```python
from build123d import *

# Parameters (mm, degrees)
SKETCH2_W  = 5.6
SKETCH2_H  = 1
SLOT_DEPTH = 0.7


with BuildPart() as part:
    # BodySke → Base-Revolve (revolve)
    with BuildSketch(Plane.XY):
        with BuildLine():
            Line((2.4, 1.5), (2.4, 2.8))
            Line((2.4, 2.8), (1.2, 2.8))
            ThreePointArc((1.2, 2.8), (0.351471863, 2.448528137), (0, 1.6))
            Line((0, 1.6), (0, 0))
            Line((0, 0), (8.4, 0))
            Line((8.4, 0), (8.4, 1.5))
            Line((8.4, 1.5), (2.4, 1.5))
        make_face()
    revolve(axis=Axis((-25.4, 0, 0), (1, 0, 0)))

    # Sketch2 → Slot (cut)
    with BuildSketch(Plane(origin=(0, 0, 0), x_dir=(0, 0, -1), z_dir=(1, 0, 0))):
        Rectangle(SKETCH2_W, SKETCH2_H)
    extrude(amount=SLOT_DEPTH, mode=Mode.SUBTRACT)


solid = part.part
```
Here's how the part is built. I have some questions about the finished solid (model axes, mm). A direction names the side the tool comes from. Round coordinates to 2 decimals unless told otherwise and drop trailing zeros. Loops run counter-clockwise (first coordinate to the right, second up) from the corner with the lowest first, then second, coordinate; pieces in that order, holes last.
1. Will these pins go through, and if not, where does the flat tip stop? pin 1 (2 mm diameter, centred on x = 3.5, z = 1, fed in from +Y); pin 2 (1.5 mm diameter, centred on y = -2, z = -1.5, fed in from +X); pin 3 (0.5 mm diameter, centred on y = 0, z = 1, fed in from -X).
Answers:
pin 1: stops at y = 1.5
pin 2: stops at x = 2.4
pin 3: stops at x = 0.7
2. Thinking about a two-plate mould opening in Y: for faces 1 (the face through (0, 1, 0)), 2 (the face through (1.8, -2.8, 0.1)), 3 (the face through (0.7, 0, 0)), which applies, released by +Y, released by -Y, zero draft, split by the parting line, or undercut?
Answers:
face 1: zero draft
face 2: split by the parting line
face 3: undercut
3. Suppose I cut it at B-B, the plane y = 0. Please give me the cut outline in (x, z).
Answers:
outline: (0.7, -2.69) arc R1.2 ccw to (1.2, -2.8) - (2.4, -2.8) - (2.4, -1.5) - (8.4, -1.5) - (8.4, 1.5) - (2.4, 1.5) - (2.4, 2.8) - (1.2, 2.8) arc R1.2 ccw to (0.7, 2.69) - close
4. For faces 4 (the face through (0, -1, 0)), 5 (the face through (5.36, -1.5, 0.07)), which set-ups out of +Z, -Z, +X, -X, +Y, -Y let a thin tool reach every point of the face, with its end or its side?
Answers:
face 4: +Z, -Z, -X, +Y, -Y
face 5: +X
5. Suppose I cut it at A-A, the plane z = 0. Please give me the cut outline in (x, y), and give its area (3 significant figures).
Answers:
outline: (0, -1.6) arc R1.2 ccw to (1.2, -2.8) - (2.4, -2.8) - (2.4, -1.5) - (8.4, -1.5) - (8.4, 1.5) - (2.4, 1.5) - (2.4, 2.8) - (1.2, 2.8) arc R1.2 ccw to (0, 1.6) - (0, 0.5) - (0.7, 0.5) - (0.7, -0.5) - (0, -0.5) - close
area: 30.1 mm2
6. If I drill on probe 1 along X at (y, z) = (-1.5, -0.65); probe 2 along X at (y, z) = (0.2, -0.2); probe 3 along Y at (x, z) = (2, 2.4), over which ranges is the centre line in solid material (lowest first)?
Answers:
probe 1: x = 0 to 2.4
probe 2: x = 0.7 to 8.4
probe 3: y = -1.44 to 1.44
7. Suppose I cut it at C-C, the plane x = 6.25. Please give me the cut outline in (y, z), and give its area (3 significant figures).
Answers:
outline: circle Ø3 at (0, 0)
area: 7.07 mm2
